Could you check a few things on this model? Use its own coordinates, in mm. Give positions to 0.01 mm unless a question says otherwise; leave off trailing zeros. Write each loop counter-clockwise with the first axis right and the second up, starting at its lowest first coordinate (ties: lowest second). Pieces come first, ordered by that corner, then holes. Notation, with made-up numbers: (11.25, 6) - (15.25, 6) arc R23 cw to (15.25, 32) - close; hole circle Ø6 at (75, 28.25). An arc over 180 degrees is marked (long way). Write item = value, one per line.
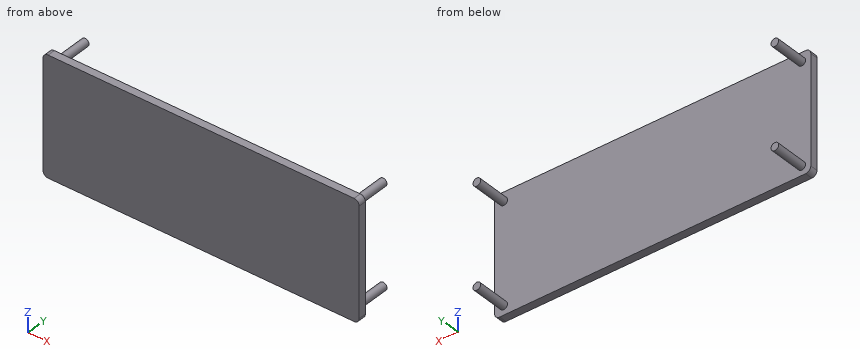
Autodesk Fusion 360 part; units mm, degrees
sketch "Sketch1" plane through (0, 0, 0) normal (0, 1, 0) x (1, 0, 0)
  line L0 (0, 0) -> (-123, 0)
  line L1 (-123, 0) -> (-123, 45.95)
  line L2 (-123, 45.95) -> (0, 45.95)
  line L3 (0, 45.95) -> (0, 0)
  dimension "d1" = 123
  dimension "d2" = 45.95
extrude "Extrude1" add sketch "Sketch1" along normal blind 3
sketch "Sketch2" plane through (0, 3, 0) normal (0, 1, 0) x (-1, 0, 0)
  line L0 (0, -45.95) -> (123, -45.95)
  line L1 (123, -45.95) -> (123, 0)
  line L2 (123, 0) -> (0, 0)
  line L3 (0, 0) -> (0, -45.95)
  line L4 (0, 0) -> (5, 0) construction
  line L5 (123, 0) -> (128, 0) construction
  line L6 (123, -45.95) -> (128, -45.95) construction
  line L7 (0, -45.95) -> (5, -45.95) construction
  circle A0 centre (119.4645, -42.4145) radius 1.5
  circle A1 centre (3.5355, -42.4145) radius 1.5
  circle A2 centre (119.4645, -3.5355) radius 1.5
  circle A3 centre (3.5355, -3.5355) radius 1.5
  dimension "d5" = 5
  dimension "d8" = 5
  dimension "d10" = 5
  dimension "d11" = 5
  dimension "d13" = 3
  dimension "d14" = 3
  dimension "d15" = 3
  dimension "d16" = 3
extrude "Extrude2" add sketch "Sketch2" along normal blind 13 contours A0 | A1 | A2 | A3
fillet "Fillet1" radius 2 2 edges at (-123, 1.5, 0) (0, 1.5, 0)
fillet "Fillet2" radius 2 2 edges at (0, 1.5, -45.95) (-123, 1.5, -45.95)
1. If we section it at A-A, the plane z = -35: Please give me the cut outline in (x, y), and give its area (3 significant figures).
Filled sheet:
outline = (-123, 0) - (0, 0) - (0, 3) - (-123, 3) - close
area = 369 mm2
2. I need wall thicknesses on line 1 (Y direction, x = -84.5, z = -34.5); line 2 (X direction, y = 4.75, z = -43). Which ranges of each line are inside material? Lowest first, please.
Filled sheet:
line_1 = 0 to 3
line_2 = -120.85 to -118.08, -4.92 to -2.15
3. For pin 1 (10 mm diameter, centred on x = -60, z = -22.5, fed in from +Y); pin 2 (8 mm diameter, centred on x = -77.5, y = 8.5, fed in from +Z), each with a flat end and sliding along its axis, tell me the tip position at first contact or that it passes through.
Filled sheet:
pin_1 = 3
pin_2 = through
4. If we section it at C-C, the plane y = 14: Please give me the cut outline in (x, z), and give its area (3 significant figures).
Filled sheet:
outline = circle Ø3 at (-119.46, -42.41); circle Ø3 at (-119.46, -3.54); circle Ø3 at (-3.54, -42.41); circle Ø3 at (-3.54, -3.54)
area = 28.3 mm2
5. If we section it at B-B, the plane x = -114: Please give me the cut outline in (y, z), and give its area (3 significant figures).
Filled sheet:
outline = (0, -45.95) - (3, -45.95) - (3, 0) - (0, 0) - close
area = 138 mm2
